Autodesk Inventor part; units mm, degrees
ref_plane "YZ Plane" through (0, 0, 0) normal (1, 0, 0) x (0, 1, 0)
ref_plane "XZ Plane" through (0, 0, 0) normal (0, 1, 0) x (-1, 0, 0)
ref_plane "XY Plane" through (0, 0, 0) normal (0, 0, 1) x (1, 0, 0)
sketch "Sketch1" plane through (0, 0, 0) normal (0, 1, 0) x (-1, 0, 0)
  circle A0 centre (0, 0) radius 62.865
  circle A1 centre (0, 0) radius 69.85
  circle A2 centre (0, 0) radius 64.4525
  dimension "d0" = 125.73
  dimension "d1" = 139.7
  dimension "d2" = 1.5875
extrude "Extrusion1" add sketch "Sketch1" along normal blind 28.575 contours A2
extrude "Extrusion2" add sketch "Sketch1" along normal blind 3.175 contours A1
chamfer "Chamfer1" distance 2.54 angle 45 1 edges at (69.85, 0, 0)
properties part number "Bevel V1_3DPrint"
Build history of the part. All positions in model axes, mm. A direction names the side the tool comes from. Round coordinates to 2 decimals unless told otherwise and drop trailing zeros. Loops run counter-clockwise (first coordinate to the right, second up) from the corner with the lowest first, then second, coordinate; pieces in that order, holes last. Notation, with made-up numbers: (73.5, 10) -> (126.5, 10) arc R21 cw to (126.5, 14) -> close; hole circle Ø2 at (77, -28.5). An arc over 180 degrees is marked (long way). Use CSV: the item, a comma, the result in double quotes. Start each with the question number.
Q1. Which spindle directions (+Z, -Z, +X, -X, +Y, -Y) get a long thin tool onto all of the face, cutting with end or side? Do faces 4 (the face through (55.431, 2.853, 42.503)), 5 (the face through (64.39, 15.7, -2.83)). Say none if no direction does.
Q2. Mould opens along X. For faces 1 (the face through (8.783, 0.159, 66.895)), 2 (the face through (-20, 3.175, -62)), 3 (the face through (49.89, 14.09, 38.25)) say: +X half, -X half, draft (parallel to the pull), parting line (faces both ways), or undercut.
Q3. Drill centre lines: L1, parallel to Z at x = 0, y = 12.5 (1 decimal); L2, parallel to Y at x = 37.5, z = 55 (3 decimals); L3, parallel to Z at x = 55.5, y = 21. Where is each one in solid material? Low to high.
Q4. Flat gauge pins, fed straight in: pin 1 Ø4 at (y, z) = (11.5, -8) entering from -X; pin 2 Ø2 at (y, z) = (25.5, -5.5) entering from -X; pin 3 Ø1 at (x, y) = (-47.5, 6.5) entering from +Z. Where does each tip first touch, or does it go through?
Q5. Saw through at C-C on y = 23.75. Give the cut face in (x, z) (1 decimal), and give its area (3 significant figures).
Solutions:
1,face 4,"+Y, -Y"
1,face 5,"+Y"
2,face 1,"parting line"
2,face 2,"draft"
2,face 3,"undercut"
3,L1,"z = -64.5 to -62.9, 62.9 to 64.5"
3,L2,"y = 0 to 3.175"
3,L3,"z = -32.77 to -29.53, 29.53 to 32.77"
4,pin 1,"stops at x = -64.17"
4,pin 2,"stops at x = -64.3"
4,pin 3,"stops at z = 44.1"
5,outline,"circle Ø128.9 at (0, 0); hole circle Ø125.7 at (0, 0)"
5,area,"635 mm^2"
